Verification items for the finished model (mm, model axes). Coordinates: 2 decimals unless noted, no trailing zeros. Loops run counter-clockwise (first coordinate to the right, second up) from the corner with the lowest first, then second, coordinate; pieces in that order, holes last. Notation, with made-up numbers: (81, 37.5) - (98, 37.5) arc R16 ccw to (98, 48.5) - close; hole circle Ø2 at (27.5, 17.5). An arc over 180 degrees is marked (long way). Answer as CSV lines item,"result". Start each with the question number.
1. Gauge pin test, flat ends, axial feed: P1, Ø11.5, axis at x = 0, z = 52, coming from the +Y side; P2, Ø8, axis at x = -52, z = 0, coming from the -Y side; P3, Ø1, axis at x = -50, y = 4, coming from the +Z side. Record the tip position at first contact, or that the pin passes through.
2. Release check for a two-part mould opening along X. For faces 1 (the flat face through (-1, 0, -16)), 2 (the cylindrical face through (-14.524, 2.465, 65.407)), 3 (the cylindrical face through (-1.86, 2.54, -14.18)) record: pulls with the +X half, pulls with the -X half, needs draft (parallel to the pull), parting line crosses it, or undercut.
3. Cross-section at C-C (x = -52). Enter the section's corners in (y, z).
4. Material ranges on line 1 (Z direction, x = 0, y = 3.75); line 2 (X direction, y = 3.55, z = 4), recorded low to high. Write a range as [from, to].
5. Cross-section at D-D (y = 2). Enter the section's corners in (x, z), plus the area to 3 significant figures.
6. Cross-section at A-A (z = 0). Enter the section's corners in (x, y), plus the area to 3 significant figures.
7. Cross-section at B-B (x = 0). Enter the section's corners in (y, z), plus the area to 3 significant figures.
```python
from build123d import *

# Parameters (mm, degrees)
SKETCH1_R               = 67
SKETCH1_R_2             = 5
BOSS_EXTRUDE1_DEPTH     = 5
SKETCH2_4_R             = 14.3
CUT_EXTRUDE3_DEPTH      = 1
CUT_EXTRUDE3_DEPTH_BACK = 6


with BuildPart() as part:
    # Sketch1 → Boss-Extrude1 (new body)
    with BuildSketch(Plane(origin=(0, 0, 0), x_dir=(1, 0, 0), z_dir=(0, 1, 0))):
        Circle(SKETCH1_R)
        with Locations((0, 52)):
            Circle(SKETCH1_R_2, mode=Mode.SUBTRACT)
        with Locations((52, 0)):
            Circle(SKETCH1_R_2, mode=Mode.SUBTRACT)
        with Locations((0, -52)):
            Circle(SKETCH1_R_2, mode=Mode.SUBTRACT)
        with Locations((-52, 0)):
            Circle(SKETCH1_R_2, mode=Mode.SUBTRACT)
    extrude(amount=BOSS_EXTRUDE1_DEPTH)

    # Sketch2<4> → Cut-Extrude3 (cut, two sides)
    with BuildSketch(Plane(origin=(0, 5, 0), x_dir=(1, 0, 0), z_dir=(0, 1, 0))) as cut_extrude3_sk:
        Circle(SKETCH2_4_R)
    extrude(amount=CUT_EXTRUDE3_DEPTH, mode=Mode.SUBTRACT)
    extrude(cut_extrude3_sk.sketch, amount=-CUT_EXTRUDE3_DEPTH_BACK, mode=Mode.SUBTRACT)


solid = part.part
```
Values follow:
1,P1,"stops at y = 5"
1,P2,"passes through"
1,P3,"stops at z = 45.15"
2,face 1,"needs draft"
2,face 2,"parting line crosses it"
2,face 3,"undercut"
3,outline,"(0, -42.25) - (5, -42.25) - (5, -5) - (0, -5) - close; (0, 5) - (5, 5) - (5, 42.25) - (0, 42.25) - close"
4,line 1,"z = [-67, -57], [-47, -14.3], [14.3, 47], [57, 67]"
4,line 2,"x = [-66.88, -55], [-49, -13.73], [13.73, 49], [55, 66.88]"
5,outline,"circle Ø134 at (0, 0); hole circle Ø10 at (-52, 0); hole circle Ø28.6 at (0, 0); hole circle Ø10 at (0, -52); hole circle Ø10 at (0, 52); hole circle Ø10 at (52, 0)"
5,area,"13,100 mm²"
6,outline,"(-67, 0) - (-57, 0) - (-57, 5) - (-67, 5) - close; (-47, 0) - (-14.3, 0) - (-14.3, 5) - (-47, 5) - close; (14.3, 0) - (47, 0) - (47, 5) - (14.3, 5) - close; (57, 0) - (67, 0) - (67, 5) - (57, 5) - close"
6,area,"427 mm²"
7,outline,"(0, -67) - (5, -67) - (5, -57) - (0, -57) - close; (0, -47) - (5, -47) - (5, -14.3) - (0, -14.3) - close; (0, 14.3) - (5, 14.3) - (5, 47) - (0, 47) - close; (0, 57) - (5, 57) - (5, 67) - (0, 67) - close"
7,area,"427 mm²"
